Autodesk Inventor part; units mm, degrees
ref_plane "YZ Plane" through (0, 0, 0) normal (1, 0, 0) x (0, 1, 0)
ref_plane "XZ Plane" through (0, 0, 0) normal (0, 1, 0) x (-1, 0, 0)
ref_plane "XY Plane" through (0, 0, 0) normal (0, 0, 1) x (1, 0, 0)
sketch "Sketch1" plane through (0, 0, 0) normal (0, 1, 0) x (-1, 0, 0)
  line L0 (0, 0) -> (27.3, 0)
  line L1 (27.3, 0) -> (27.3, -30.7)
  line L2 (27.3, -30.7) -> (0, -30.7)
  line L3 (0, -30.7) -> (0, 0)
  dimension "d0" = 27.3
  dimension "d1" = 30.7
extrude "Extrusion1" add sketch "Sketch1" along normal blind 31.3
sketch "Sketch2" plane through (0, 31.3, 0) normal (0, 1, 0) x (1, 0, 0)
  line L0 (-27.3, 0) -> (0, 0) construction
  line L1 (0, 0) -> (0, 7.7) construction
  line L2 (-6.5, 7.7) -> (6.5, 7.7)
  line L3 (6.5, 7.7) -> (6.5, 22.7)
  line L4 (6.5, 22.7) -> (-6.5, 22.7)
  line L5 (-6.5, 22.7) -> (-6.5, 7.7)
  dimension "d4" = 7.7
  dimension "d5" = 13
  dimension "d6" = 15
extrude "Extrusion2" add sketch "Sketch2" along normal blind 20 and the other way blind 5
draft "FaceDraft1" angle 60 pull direction (1, 0, 0) faces at (2.1667, 26.3, -17.7) fixed edges at (6.5, 26.3, -15.2)
sketch "Sketch3" plane through (-6.5, 31.3, -7.7) normal (0, 0, 1) x (1, 0, 0)
  line L0 (6.5, 0) -> (0, 0) construction
  line L1 (0, 0) -> (0, 6.2) construction
  line L2 (0, 20) -> (0, 0) construction
  line L3 (0, 6.2) -> (12.9928, 6.2) construction
  circle A0 centre (6.4964, 9.425) radius 3.225
  line L4 (0, 20) -> (13, 20)
  line L5 (0, 20) -> (13, 20)
  line L6 (13, 20) -> (13, 17.5)
  line L7 (13, 17.5) -> (0, 17.5)
  line L8 (0, 17.5) -> (0, 20)
  point P0 (6.5, -31.3)
  point P1 (6.4964, 6.2)
  dimension "d13" = 6.45
  dimension "d12" = 6.2
  dimension "d14" = 2.5
extrude "Extrusion3" cut sketch "Sketch3" against normal through all
sketch "Sketch4" plane through (0, 0, -30.7) normal (0, 0, -1) x (-1, 0, 0)
  line L0 (27.3, 31.3) -> (0, 31.3) construction
  line L1 (27.3, 31.3) -> (27.3, 19.8) construction
  line L2 (27.3, 0) -> (27.3, 31.3) construction
  line L3 (27.3, 19.8) -> (32.3, 19.8)
  line L4 (32.3, 19.8) -> (32.3, 12.8)
  line L5 (32.3, 12.8) -> (27.3, 12.8)
  line L6 (27.3, 12.8) -> (27.3, 19.8)
  point P0 (0, 0)
  dimension "d17" = 11.5
  dimension "d18" = 5
  dimension "d19" = 7
extrude "Extrusion4" add sketch "Sketch4" along normal blind 20 and the other way blind 12
draft "FaceDraft2" angle 45 pull direction (-1, 0, 0) faces at (-30.6333, 15.1333, -18.7) fixed edges at (-27.3, 16.3, -18.7)
sketch "Sketch5" plane through (0, 0, -30.7) normal (0, 0, -1) x (-1, 0, 0)
  line L0 (27.3, 19.8) -> (27.3, 31.3)
  line L1 (27.3, 31.3) -> (12.3, 31.3)
  line L2 (12.3, 31.3) -> (12.3, 24.3)
  line L3 (12.3, 24.3) -> (27.3, 24.3)
  line L4 (27.3, 24.3) -> (27.3, 31.3)
  point P0 (0, 0)
  dimension "d25" = 15
  dimension "d26" = 7
extrude "Extrusion5" cut sketch "Sketch5" against normal through all
sketch "Sketch6" plane through (0, 0, -30.7) normal (0, 0, -1) x (-1, 0, 0)
  point P0 (0, 0)
sketch "Sketch7" plane through (0, 0, -30.7) normal (0, 0, -1) x (-1, 0, 0)
  point P0 (0, 0)
sketch "Sketch8" plane through (0, 0, -30.7) normal (0, 0, -1) x (-1, 0, 0)
  line L0 (27.3, 0) -> (0, 0)
  line L1 (27.3, 0) -> (21.3, 0)
  line L2 (21.3, 0) -> (21.3, -5)
  line L3 (21.3, -5) -> (27.3, -5)
  line L4 (27.3, -5) -> (27.3, 0)
  line L5 (0, 0) -> (6, 0)
  line L6 (6, 0) -> (6, -5)
  line L7 (6, -5) -> (0, -5)
  line L8 (0, -5) -> (0, 0)
  dimension "d29" = 6
  dimension "d30" = 5
  dimension "d31" = 6
  dimension "d32" = 5
extrude "Extrusion6" add sketch "Sketch8" along normal blind 20 and the other way blind 25
draft "FaceDraft3" angle 45 pull direction (0, -1, 0) faces at (-23.3, -3.3333, -5.7) (-2, -1.6667, -5.7) fixed edges at (-24.3, 0, -5.7) (-3, 0, -5.7)
properties part number "Y- motor carrier"
Could you check a few things on this model? Use its own coordinates, in mm. A direction names the side the tool comes from. Give positions to 0.01 mm unless a question says otherwise; leave off trailing zeros. Order: outer loops, then holes, each group sorted by start corner. A loop starts at its lowest first (then second) coordinate and runs counter-clockwise, first axis right, second up.
Q1. Suppose I cut it at A-A, the plane z = -42. Write out the boundary of the cut face in (x, y).
Q2. I'm going to push flat-ended pins straight in: P1, Ø12, axis at x = -27, y = 17.5, coming from the +Z side; P2, Ø1.5, axis at y = -1.5, z = -36, coming from the +X side; P3, Ø6.5, axis at x = 0.5, y = 35.5, coming from the -Z side; P4, Ø7.5, axis at y = 37.5, z = -16, coming from the -X side. Where does each tip first touch, or does it pass through?
Q3. Suppose I cut it at B-B, the plane y = 43. Write out the boundary of the cut face in (x, z), and give its area (3 significant figures).
Q4. Suppose I cut it at D-D, the plane z = -6.5. Write out the boundary of the cut face in (x, y).
Q5. For faces 5 (the flat face through (-3, 0, -41)), 6 (the flat face through (-14, 15, -30.7)), 7 (the flat face through (-6, -2, -28)), 8 (the flat face through (-6.5, 40, -15)), 9 (the flat face through (-30, 12.8, -34)), which set-ups out of +Z, -Z, +X, -X, +Y, -Y let a thin tool reach every point of the face, with its end or its side?
Q6. We'd pull the mould along X, two halves only. Please class faces 1 (the flat face through (-21.3, -2, -28)), 2 (the flat face through (-12.3, 28, -16)), 3 (the flat face through (3.205, 20.592, -15.305)), 4 (the flat face through (0, 35, -7.7)): +X half, -X half, draft (parallel to the pull), parting line (faces both ways), or undercut.
Q7. If I drill on line 1 along Y through (x, z) = (-12, -13.5); line 2 along Z through (x, y) = (-13, 4.5); line 3 along X through (y, z) = (29.5, -9.5), over which ranges is the centre line in solid material (lowest first)?
Q8. Suppose I cut it at C-C, the plane x = 1.5. Write out the boundary of the cut face in (y, z), and give its area (3 significant figures).
Solution:
1. outline: (-32.3, 12.8) - (-27.3, 12.8) - (-27.3, 19.8) - (-32.3, 19.8) - close; (-27.3, -5) - (-21.3, -5) - (-21.3, 0) - (-27.3, 0) - close; (-6, -5) - (0, -5) - (0, 0) - (-6, 0) - close
2. P1: stops at z = 0
2. P2: stops at x = 0
2. P3: stops at z = -22.7
2. P4: stops at x = -6.5
3. outline: (-6.5, -22.7) - (-2.29, -22.7) - (-2.29, -7.7) - (-6.5, -7.7) - close; (2.28, -22.7) - (6.5, -22.7) - (6.5, -7.7) - (2.28, -7.7) - close
3. area: 126 mm2
4. outline: (-27.3, -0.8) - (-21.3, -0.8) - (-21.3, 0) - (-6, 0) - (-6, -0.8) - (0, -0.8) - (0, 31.3) - (-12.3, 31.3) - (-12.3, 24.3) - (-27.3, 24.3) - close
5. face 5: -Z, +X, -X, +Y
5. face 6: -Z, +X, +Y
5. face 7: +Z, -Z, -Y
5. face 8: +Z, -Z, -X, +Y
5. face 9: +Z, -Z, -X, -Y
6. face 1: undercut
6. face 2: -X half
6. face 3: +X half
6. face 4: draft
7. line 1: y = 0 to 31.3
7. line 2: z = -30.7 to 0
7. line 3: x = -12.3 to 6.5
8. outline: (17.64, -22.7) - (37.87, -22.7) - (37.87, -7.7) - (17.64, -7.7) - close; (43.58, -22.7) - (48.8, -22.7) - (48.8, -7.7) - (43.58, -7.7) - close
8. area: 382 mm2
